from build123d import *

# Parameters (mm, degrees)
BOSS_EXTRUDE1_DEPTH      = 1.5875
BOSS_EXTRUDE1_DEPTH_BACK = 1.5875
FILLET1_R                = 1.524
BOSS_EXTRUDE2_DEPTH      = 0.89581
BOSS_EXTRUDE2_DEPTH_BACK = 0.89581
FILLET2_R                = 1.016


with BuildPart() as part:
    # Sketch1 → Boss-Extrude1 (new, two sides: drawn at the far end of the back side and taken through both)
    with BuildSketch(Plane(origin=(0, 0, 0), x_dir=(1, 0, 0), z_dir=(0, 1, 0)).offset(-BOSS_EXTRUDE1_DEPTH_BACK)):
        with BuildLine():
            Line((-0.068296764, 6.214618695), (-0.068296764, 13.138711739))
            Line((-0.068296764, 13.138711739), (-0.895808533, 13.138711739))
            add(Edge.make_bspline(
                [(-0.895808533, 13.138711739), (-1.210074473, 4.57087153), (-2.777608758, 1.083562638), (-3.277136157, 0.201945645), (0, -1.169953638)],
                knots=[0, 0, 0, 0, 0, 1, 1, 1, 1, 1], degree=4))
            add(Edge.make_bspline(
                [(0.895808533, 13.138711739), (1.210074473, 4.57087153), (2.777608758, 1.083562638), (3.277136157, 0.201945645), (0, -1.169953638)],
                knots=[0, 0, 0, 0, 0, 1, 1, 1, 1, 1], degree=4))
            Line((0.895808533, 13.138711739), (0.068296764, 13.138711739))
            Line((0.068296764, 13.138711739), (0.068296764, 6.214618695))
            add(Edge.make_bspline(
                [(1.054098961, 2.89573812), (0.161537854, 3.688347072), (0.068296764, 6.214618695)],
                knots=[0, 0, 0, 1, 1, 1], degree=2))
            ThreePointArc((1.054098961, 2.89573812), (0, 0.121211739), (-1.054098961, 2.89573812))
            add(Edge.make_bspline(
                [(-1.054098961, 2.89573812), (-0.161537854, 3.688347072), (-0.068296764, 6.214618695)],
                knots=[0, 0, 0, 1, 1, 1], degree=2))
        make_face()
    extrude(amount=BOSS_EXTRUDE1_DEPTH + BOSS_EXTRUDE1_DEPTH_BACK)

    # Fillet1
    fillet1_edges = [part.edges().sort_by_distance(p)[0] for p in [
        (0, -0.79375, 1.169953638),
    ]]
    fillet(fillet1_edges, radius=FILLET1_R)

    # Sketch2 → Boss-Extrude2 (add, two sides: drawn at the far end of the back side and taken through both)
    with BuildSketch(Plane(origin=(0, 0, 0), x_dir=(0, 0, -1), z_dir=(1, 0, 0)).offset(-BOSS_EXTRUDE2_DEPTH_BACK)):
        Polygon((13.138711739, 1.5875), (13.138711739, -1.5875), (13.138711739, -23.8125), (14.154711739, -23.8125), (14.154711739, 1.5875), align=None)
    extrude(amount=BOSS_EXTRUDE2_DEPTH + BOSS_EXTRUDE2_DEPTH_BACK)

    # Fillet2
    fillet2_edges = [part.edges().sort_by_distance(p)[0] for p in [
        (0, 1.5875, -14.154711739),
        (0.482052648, -1.5875, -13.138711739),
        (-0.482052648, -1.5875, -13.138711739),
    ]]
    fillet(fillet2_edges, radius=FILLET2_R - 0.0001)  # a hair under: the kernel refuses the full size


solid = part.part
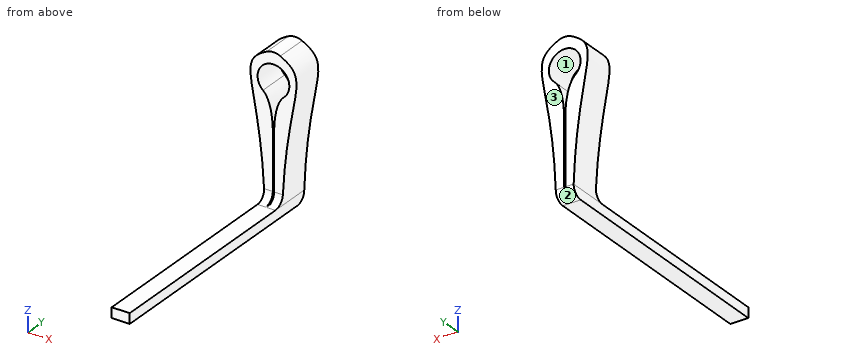
Model file for the job. Use its own axes, mm. Face numbers are marked on the shaded views. Give positions to 0.01 mm unless a question says otherwise; leave off trailing zeros. Write each loop counter-clockwise with the first axis right and the second up, starting at its lowest first coordinate (ties: lowest second). Pieces come first, ordered by that corner, then holes. Notation, with made-up numbers: M 44.5,-5.5 L 56.5,-5.5 A18 ccw 56.5,3.5 Z; hole C 1.25,46.25 d5. An arc over 180 degrees is marked long. One line per item, written item: value. Start each with the question number.
Q1. Saw through at A-A, the plane y = -4.5. Write the cut outline in (x, z).
Q2. Drop flat-ended pins along their axis: pin 1 Ø0.8 at (y, z) = (-6.5, -13.5) entering from -X; pin 2 Ø2 at (x, z) = (-0.5, -5) entering from -Y; pin 3 Ø4.5 at (y, z) = (-1, -9) entering from +X. Give the stop position or say it passes through.
Q3. Two-plate mould, pull along Z, no slides. Class the marked faces 1, 2 and 3: +Z half, -Z half, draft (parallel to the pull), parting line (faces both ways), or undercut.
Q4. Probe probe 1 along Z at (x, y) = (0, 0); probe 2 along Y at (x, z) = (0.55, -10); probe 3 along Z at (x, y) = (0.6, -3). List the from-to ranges inside material, lowest first. Write a range as [from, to].
Output values:
1. outline: M -0.9,-14.15 L 0.9,-14.15 L 0.9,-13.14 L -0.9,-13.14 Z
2. pin 1: stops at x = -0.9
2. pin 2: stops at y = -1.59
2. pin 3: stops at x = 1.47
3. face 1: undercut
3. face 2: -Z half
3. face 3: draft
4. probe 1: z = [-14.15, -13.14], [-0.12, 1.02]
4. probe 2: y = [-1.59, 1.59]
4. probe 3: z = [-14.15, -13.14]
